Verification items for the finished model (mm, model axes). Give positions to 0.01 mm unless a question says otherwise; leave off trailing zeros. Write each loop counter-clockwise with the first axis right and the second up, starting at its lowest first coordinate (ties: lowest second). Pieces come first, ordered by that corner, then holes.
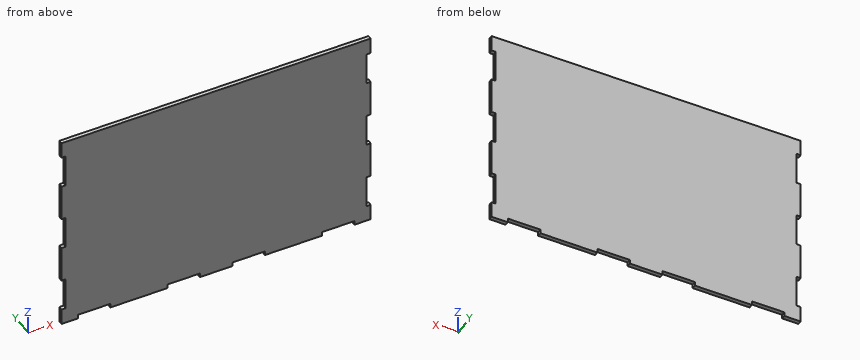
from build123d import *

# Parameters (mm, degrees)
F1_DEPTH = 3.175


with BuildPart() as f1:
    # F0 (on Front) → F1 (new body)
    with BuildSketch(Plane.XZ):
        Polygon((107.95, -79.375), (120.65, -79.375), (120.65, -66.675), (117.475, -66.675), (117.475, -41.275), (120.65, -41.275), (120.65, -12.7), (117.475, -12.7), (117.475, 0), (117.475, 12.7), (120.65, 12.7), (120.65, 41.275), (117.475, 41.275), (117.475, 66.675), (120.65, 66.675), (120.65, 79.375), (-120.65, 79.375), (-120.65, 66.675), (-117.475, 66.675), (-117.475, 41.275), (-120.65, 41.275), (-120.65, 12.7), (-117.475, 12.7), (-117.475, 0), (-117.475, -12.7), (-120.65, -12.7), (-120.65, -41.275), (-117.475, -41.275), (-117.475, -66.675), (-120.65, -66.675), (-120.65, -79.375), (-107.95, -79.375), (-107.95, -76.2), (-82.55, -76.2), (-82.55, -79.375), (-38.1, -79.375), (-38.1, -76.2), (-12.7, -76.2), (-12.7, -79.375), (12.7, -79.375), (12.7, -76.2), (38.1, -76.2), (38.1, -79.375), (82.55, -79.375), (82.55, -76.2), (107.95, -76.2), align=None)
    extrude(amount=F1_DEPTH)


solid = f1.part
Item 1: Depth check by flat-ended pin: pin 1 (1 mm diameter, centred on y = -2.5, z = 3, fed in from -X) (3 decimals); pin 2 (1 mm diameter, centred on x = 100.5, y = -1, fed in from -Z). Enter the tip coordinate at first touch or a pass-through.
Answer key:
pin 1: stops at x = -117.475
pin 2: stops at z = -76.2
Item 2: Sectioned sample at A-A on x = -90. Record the cut outline in (y, z) (3 decimals).
Answer key:
outline: (-3.175, -76.2) - (0, -76.2) - (0, 79.375) - (-3.175, 79.375) - close
Item 3: Scan lines: line 1 along Z through (x, y) = (102, -2.4) (3 decimals); line 2 along X through (y, z) = (-1.55, -48.5) (3 decimals). Record each from-to range of solid material in increasing order.
Answer key:
line 1: z = -76.2 to 79.375
line 2: x = -117.475 to 117.475
Item 4: Sectioned sample at B-B on z = 6. Record the cut outline in (x, y) (3 decimals).
Answer key:
outline: (-117.475, -3.175) - (117.475, -3.175) - (117.475, 0) - (-117.475, 0) - close
